Geometry check sheet. Reference: the model listing, model coordinates, mm. A direction names the side the tool comes from. Round coordinates to 2 decimals unless told otherwise and drop trailing zeros. Loops run counter-clockwise (first coordinate to the right, second up) from the corner with the lowest first, then second, coordinate; pieces in that order, holes last. Notation, with made-up numbers: (46.25, -39) - (63.25, -39) arc R27 cw to (63.25, -20) - close; hole circle Ø3 at (25, 21.5). An arc over 180 degrees is marked (long way). Answer as CSV lines item,"result". Start each with the question number.
1) Access from +Z, -Z, +X, -X, +Y, -Y to the whole of each face (thin tool, end or side, straight path). Record for faces 4 (the flat face through (1, 0, 0)), 5 (the flat face through (10.25, 0, 3)).
2) Cross-section at A-A on x = 25. Record the boundary of the cut face in (y, z).
3) Cross-section at B-B on z = 4. Record the boundary of the cut face in (x, y).
4) Draft check along Y on faces 1 (the flat face through (1, 24, 3)), 2 (the flat face through (42.5, 0, 3)), 3 (the flat face through (-10.25, 0, 3)). Enter one of: released by +Y, released by -Y, zero draft, split by the parting line, or undercut.
5) Thickness scan on line 1 along X through (y, z) = (-4, 3); line 2 along Y through (x, z) = (-15.5, 1.5). Record the ranges inside material, lowest first.
6) Cross-section at C-C on y = -1.5. Record the boundary of the cut face in (x, z).
from build123d import *

# Parameters (mm, degrees)
F0_W     = 42.5
F0_H     = 48
F1_DEPTH = 6.7
F2_W     = 19.5
F2_H     = 28.5
F3_DEPTH = 25
F5_SIZE  = 1.2


with BuildPart() as f1:
    # F0 (on Top) → F1 (new body)
    with BuildSketch(Plane.XY):
        with Locations((21.25, 0)):
            Rectangle(F0_W, F0_H)
    extrude(amount=F1_DEPTH)

    # F2 (on face) → F3 (cut)
    with BuildSketch(Plane.XY.offset(6.7)):
        with Locations((20, 0)):
            Rectangle(F2_W, F2_H)
    extrude(amount=-F3_DEPTH, mode=Mode.SUBTRACT)

    # F4: F1 across plane


with BuildPart() as f1_1:
    add(f1.part)
    add(f1.part.mirror(Plane.YZ))

    # F5
    f5_edges = [f1_1.edges().sort_by_distance(p)[0] for p in [
        (0, 24, 6.7),
        (-42.5, 0, 6.7),
        (0, -24, 6.7),
        (42.5, 0, 0),
        (29.75, 0, 6.7),
        (10.25, 0, 6.7),
        (-10.25, 0, 6.7),
        (-29.75, 0, 6.7),
        (-20, 14.25, 6.7),
        (-20, -14.25, 6.7),
        (20, -14.25, 6.7),
        (20, 14.25, 6.7),
        (-42.5, -24, 3.35),
        (-42.5, 0, 0),
        (-42.5, 24, 3.35),
        (0, -24, 0),
        (-20, -14.25, 0),
        (-10.25, 0, 0),
        (-20, 14.25, 0),
        (-29.75, 0, 0),
        (10.25, 0, 0),
        (29.75, 0, 0),
        (20, 14.25, 0),
        (20, -14.25, 0),
        (42.5, 24, 3.35),
        (42.5, -24, 3.35),
        (42.5, 0, 6.7),
        (0, 24, 0),
    ]]
    chamfer(f5_edges, length=F5_SIZE)


solid = f1_1.part
Answer block:
1,face 4,"-Z, +X, -X, +Y, -Y"
1,face 5,"+Z, -Z"
2,outline,"(-24, 1.2) - (-22.8, 0) - (-15.45, 0) - (-14.25, 1.2) - (-14.25, 5.5) - (-15.45, 6.7) - (-22.8, 6.7) - (-24, 5.5) - close; (14.25, 1.2) - (15.45, 0) - (22.8, 0) - (24, 1.2) - (24, 5.5) - (22.8, 6.7) - (15.45, 6.7) - (14.25, 5.5) - close"
3,outline,"(-42.5, -22.8) - (-41.3, -24) - (41.3, -24) - (42.5, -22.8) - (42.5, 22.8) - (41.3, 24) - (-41.3, 24) - (-42.5, 22.8) - close; hole (-29.75, -14.25) - (-10.25, -14.25) - (-10.25, 14.25) - (-29.75, 14.25) - close; hole (10.25, -14.25) - (29.75, -14.25) - (29.75, 14.25) - (10.25, 14.25) - close"
4,face 1,"released by +Y"
4,face 2,"zero draft"
4,face 3,"undercut"
5,line 1,"x = -42.5 to -29.75, -10.25 to 10.25, 29.75 to 42.5"
5,line 2,"y = -24 to -14.25, 14.25 to 24"
6,outline,"(-42.5, 1.2) - (-41.3, 0) - (-30.95, 0) - (-29.75, 1.2) - (-29.75, 5.5) - (-30.95, 6.7) - (-41.3, 6.7) - (-42.5, 5.5) - close; (-10.25, 1.2) - (-9.05, 0) - (9.05, 0) - (10.25, 1.2) - (10.25, 5.5) - (9.05, 6.7) - (-9.05, 6.7) - (-10.25, 5.5) - close; (29.75, 1.2) - (30.95, 0) - (41.3, 0) - (42.5, 1.2) - (42.5, 5.5) - (41.3, 6.7) - (30.95, 6.7) - (29.75, 5.5) - close"
